Geometry: final body of the model. Coordinates: model frame, mm. A direction names the side the tool comes from. Round coordinates to 2 decimals unless told otherwise and drop trailing zeros. Order: outer loops, then holes, each group sorted by start corner. A loop starts at its lowest first (then second) coordinate and runs counter-clockwise, first axis right, second up. Notation, with made-up numbers: M -29,-12.5 L 7,-12.5 A21 cw 7,17.5 Z; hole C 46.25,52.25 d1. An arc over 180 degrees is marked long. Put each result on its own line as item: value. Start each with the question number.
1) Section C-C, the plane z = 0.7. Return loops of the section in (x, y), then the cut area to 3 significant figures.
2) Section D-D, the plane z = 2.2. Return loops of the section in (x, y), then the cut area to 3 significant figures.
3) First-contact query: P1, Ø1.5, axis at y = 2.5, z = 1.5, coming from the +X side; P2, Ø5, axis at x = -3, y = 0.5, coming from the -Z side. Flat tips, straight axial feed; report the tip coordinate or a pass-through.
4) Material intervals for probe 1 along Y at (x, z) = (0, 1.6); probe 2 along X at (y, z) = (-1.75, 1.3); probe 3 along X at (y, z) = (2.25, 0.2), sorted ascending. Write a range as [from, to].
5) Access query for faces 1 (the flat face through (2.2, -3.3, 0)), 2 (the cylindrical face through (3.233, -1.341, 3.493)). Directions: +Z, -Z, +X, -X, +Y, -Y. A direction counts if a zero-diameter tool reaches every point of the face in a straight line with its end or side. Return the directions, or none.
from build123d import *

# Parameters (mm, degrees)
SKETCH1_R           = 5
BOSS_EXTRUDE1_DEPTH = 2
SKETCH2_R           = 2.5
CUT_EXTRUDE1_DEPTH  = 10
SKETCH3_R           = 3.5
BOSS_EXTRUDE2_DEPTH = 2
CUT_EXTRUDE2_START  = -3
SKETCH4_R           = 2.5
CUT_EXTRUDE2_DEPTH  = 3
FILLET1_R           = 1
FILLET2_R           = 1
FILLET3_R           = 1


with BuildPart() as part:
    # Sketch1 → Boss-Extrude1 (new body)
    with BuildSketch(Plane.XY):
        Circle(SKETCH1_R)
    extrude(amount=BOSS_EXTRUDE1_DEPTH)

    # Sketch2 → Cut-Extrude1 (cut)
    with BuildSketch(Plane.XY.offset(2)):
        Circle(SKETCH2_R)
    extrude(amount=-CUT_EXTRUDE1_DEPTH, mode=Mode.SUBTRACT)

    # Sketch3 → Boss-Extrude2 (add)
    with BuildSketch(Plane.XY.offset(2)):
        Circle(SKETCH3_R)
    extrude(amount=BOSS_EXTRUDE2_DEPTH)

    # Sketch4 → Cut-Extrude2 (cut)
    with BuildSketch(Plane(origin=(0, 0, 2), x_dir=(-1, 0, 0), z_dir=(0, 0, -1)).offset(CUT_EXTRUDE2_START)):
        with Locations(Location((0, 0, 0), (0, 0, 180))):
            Circle(SKETCH4_R)
    extrude(amount=CUT_EXTRUDE2_DEPTH, mode=Mode.SUBTRACT)

    # Fillet1
    fillet1_edges = [part.edges().sort_by_distance(p)[0] for p in [
        (-2.5, 0, 0),
    ]]
    fillet(fillet1_edges, radius=FILLET1_R)

    # Fillet2
    fillet2_edges = [part.edges().sort_by_distance(p)[0] for p in [
        (-2.5, 0, 4),
    ]]
    fillet(fillet2_edges, radius=FILLET2_R - 0.0001)  # a hair under: the kernel refuses the full size

    # Fillet3
    fillet3_edges = [part.edges().sort_by_distance(p)[0] for p in [
        (-3.5, 0, 2),
    ]]
    fillet(fillet3_edges, radius=FILLET3_R)


solid = part.part
Result sheet:
1. outline: C 0,0 d10; hole C 0,0 d5.09
1. area: 58.2 mm2
2. outline: C 0,0 d7.8; hole C 0,0 d5
2. area: 28.1 mm2
3. P1: stops at x = 4.68
3. P2: stops at z = 0
4. probe 1: y = [-5, -2.5], [2.5, 5]
4. probe 2: x = [-4.68, -1.79], [1.79, 4.68]
4. probe 3: x = [-4.47, -1.83], [1.83, 4.47]
5. face 1: -Z, +X, -X, +Y, -Y
5. face 2: +Z
